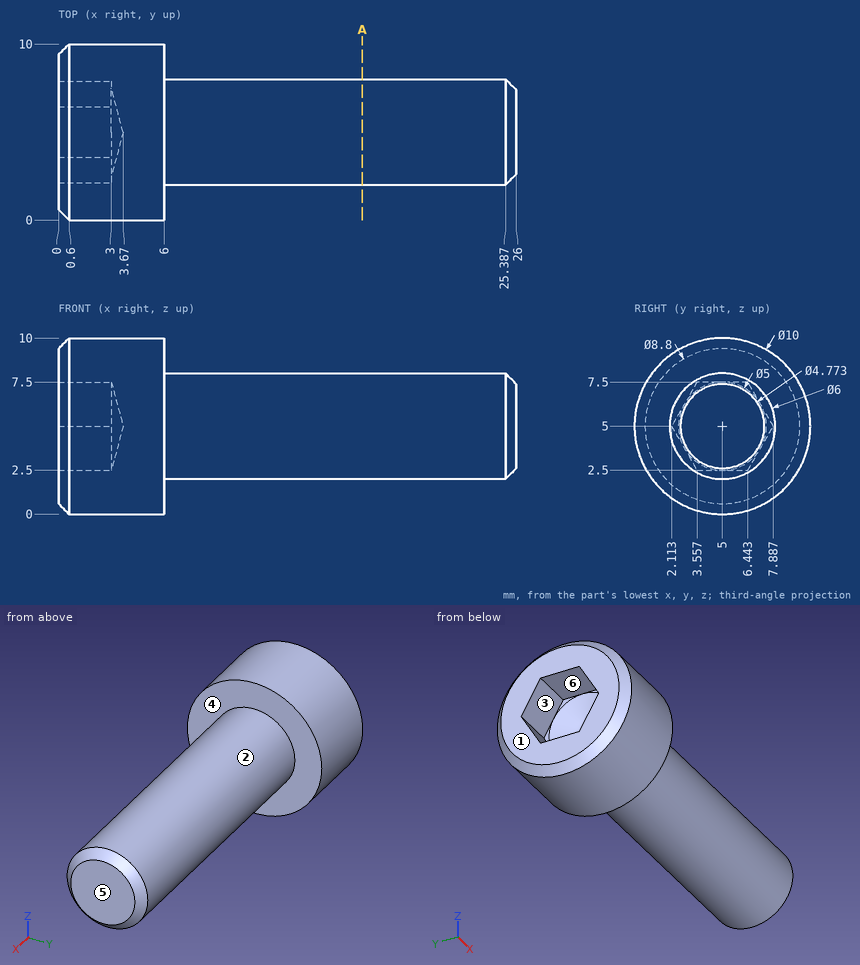
Source: three-view drawing plus pictorial views. Frame: mm from the lowest corner of the part. A direction names the side the tool comes from. Coordinates: 2 decimals unless noted, no trailing zeros. Order: outer loops, then holes, each group sorted by start corner. A loop starts at its lowest first (then second) coordinate and runs counter-clockwise, first axis right, second up.
1) Set-up query: the marked faces 4, 5 and 6. Return all of +Z, -Z, +X, -X, +Y, -Y with unobstructed straight access to the full face (end or side cutting, diameter ignored); none if empty.
Result sheet:
face 4: +X
face 5: +Z, -Z, +X, +Y, -Y
face 6: -X
2) Section A-A (x = 17.25). Return loops of the section in (y, z), then the cut area to 3 significant figures.
Result sheet:
outline: circle Ø6 at (5, 5)
area: 28.3 mm2
3) Ray query, probe 1 along X at (y, z) = (7.75, 3); probe 2 along Y at (x, z) = (2, 5.5) (1 decimal); probe 3 along Y at (x, z) = (16.5, 4). Return the intervals inside material, ascending.
Result sheet:
probe 1: x = 0 to 6
probe 2: y = 0 to 2.4, 7.6 to 10
probe 3: y = 2.17 to 7.83
4) Draft query along Z for the marked faces 1, 2 and 3. Return one class per face: released by +Z, released by -Z, zero draft, split by the parting line, or undercut.
Result sheet:
face 1: zero draft
face 2: split by the parting line
face 3: undercut
5) First-contact query: P1, Ø3, axis at x = 10, z = 6.5, coming from the +Y side; P2, Ø1, axis at x = 3.5, y = 1.5, coming from the +Z side; P3, Ø1, axis at x = 8.5, y = 6.5, coming from the +Z side. Flat tips, straight axial feed; report the tip coordinate or a pass-through.
Result sheet:
P1: stops at y = 8
P2: stops at z = 9
P3: stops at z = 7.83
